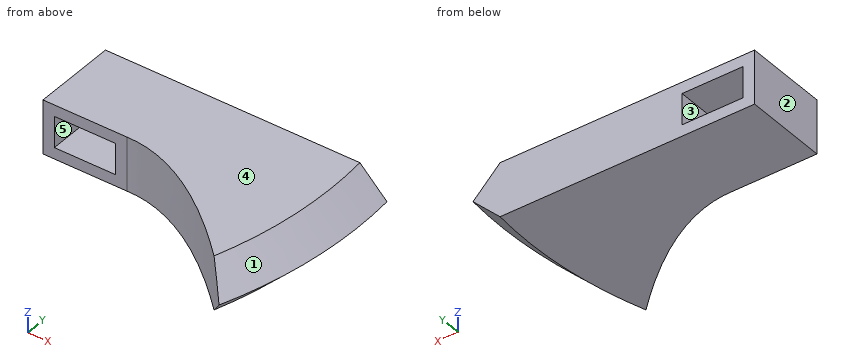
```python
from build123d import *

# Parameters (mm, degrees)
BOSS_EXTRUDE1_DEPTH     = 9
CUT_EXTRUDE1_DEPTH      = 48.981771871
CUT_EXTRUDE1_DEPTH_BACK = 48.981771871
SKETCH2_W               = 10.2
SKETCH2_H               = 5.2
CHAMFER1_SIZE           = 5


with BuildPart() as part:
    # Sketch1 → Boss-Extrude1 (new body)
    with BuildSketch(Plane.XY):
        with BuildLine():
            Line((-34.136986301, -14), (-34.136986301, -28))
            Line((-34.136986301, -28), (-20.136986301, -28))
            add(Edge.make_bspline(
                [(-20.136986301, -28), (-8.577544678, -27.582757126), (9.091518621, -46.494870104)],
                knots=[0, 0, 0, 1, 1, 1], degree=2))
            ThreePointArc((9.091518621, -46.494870104), (13.07538723, -30.490408573), (13.358976811, -14))
            Line((13.358976811, -14), (-20.136986301, -14))
            Line((-20.136986301, -14), (-34.136986301, -14))
        make_face()
    extrude(amount=BOSS_EXTRUDE1_DEPTH)

    # Sketch2 → Cut-Extrude1 (cut, two sides: drawn at the far end of the back side and taken through both)
    with BuildSketch(Plane(origin=(0, -14, 0), x_dir=(1, 0, 0), z_dir=(0, 1, 0)).offset(-CUT_EXTRUDE1_DEPTH_BACK)):
        with Locations((-27.136986301, -4.5)):
            Rectangle(SKETCH2_W, SKETCH2_H)
    extrude(amount=CUT_EXTRUDE1_DEPTH + CUT_EXTRUDE1_DEPTH_BACK, mode=Mode.SUBTRACT)

    # Chamfer1
    # the kernel refuses this chamfer: 5 mm, written as the material it takes off along each edge
    with BuildSketch(Plane(origin=(-59.190017632, -21, 0), x_dir=(0.8608936735034536, -0.5087849083077534, 0), z_dir=(-0.5087849083077534, -0.8608936735034536, 0))) as chamfer1_piece_1:
        Polygon((72.885914927 - CHAMFER1_SIZE, 0), (72.885914927, CHAMFER1_SIZE), (72.885914927, 0), align=None)
    revolve(axis=Axis((-59.190017632, -21, 0), (0, 0, 1)), revolution_arc=46.202504034, mode=Mode.SUBTRACT)
    with BuildSketch(Plane(origin=(-59.190017632, -21, 9), x_dir=(0.8608936735034536, -0.5087849083077534, 0), z_dir=(-0.5087849083077534, -0.8608936735034536, 0))) as chamfer1_piece_2:
        Polygon((72.885914927 - CHAMFER1_SIZE, 0), (72.885914927, -CHAMFER1_SIZE), (72.885914927, 0), align=None)
    revolve(axis=Axis((-59.190017632, -21, 9), (0, 0, 1)), revolution_arc=46.202504034, mode=Mode.SUBTRACT)


solid = part.part
```
Here's how the part is built. I have some questions about the finished solid (model axes, mm). Face numbers are marked on the shaded views. A direction names the side the tool comes from. Give positions to 0.01 mm unless a question says otherwise; leave off trailing zeros. Loops run counter-clockwise (first coordinate to the right, second up) from the corner with the lowest first, then second, coordinate; pieces in that order, holes last. Notation, with made-up numbers: (-12, -25.75) -> (47, -25.75) arc R17 ccw to (47, -5.75) -> close; hole circle Ø2 at (-40, -33). An arc over 180 degrees is marked (long way). Use one line per item in the form item = value. Start each with the question number.
1) Which directions (+Z, -Z, +X, -X, +Y, -Y) give clear straight access to the entire face, cutting with the end or side of a thin tool? Please do the marked faces 4 and 5.
2) Thinking about a two-plate mould opening in Z: for the marked faces 1, 2 and 3, which applies, +Z half, -Z half, draft (parallel to the pull), parting line (faces both ways), or undercut?
3) For P1, Ø2.5, axis at x = -30.5, z = 6, coming from the -Y side; P2, Ø2.5, axis at y = -23.5, z = 5, coming from the +X side; P3, Ø2, axis at y = -33.5, z = 3.5, coming from the +X side, each with a flat end and sliding along its axis, tell me the tip position at first contact or that it passes through.
4) Please list where these lines run through material, in increasing order: line 1 along Z through (x, y) = (-32, -18.5); line 2 along Y through (x, z) = (-19.5, 6); line 3 along X through (y, z) = (-21, 5.25).
5) Imagine slicing it at A-A (x = -23.5). Please give me the cut outline in (y, z).
Check values:
q1.face_4 = +Z, +X, -X, +Y, -Y
q1.face_5 = +Y, -Y
q2.face_1 = +Z half
q2.face_2 = draft
q2.face_3 = undercut
q3.P1 = -28
q3.P2 = 13.18
q3.P3 = 12.12
q4.line_1 = 0 to 1.9, 7.1 to 9
q4.line_2 = -27.99 to -14
q4.line_3 = -34.14 to -32.24, -22.04 to 12.45
q5.outline = (-28, 0) -> (-14, 0) -> (-14, 1.9) -> (-28, 1.9) -> close; (-28, 7.1) -> (-14, 7.1) -> (-14, 9) -> (-28, 9) -> close
